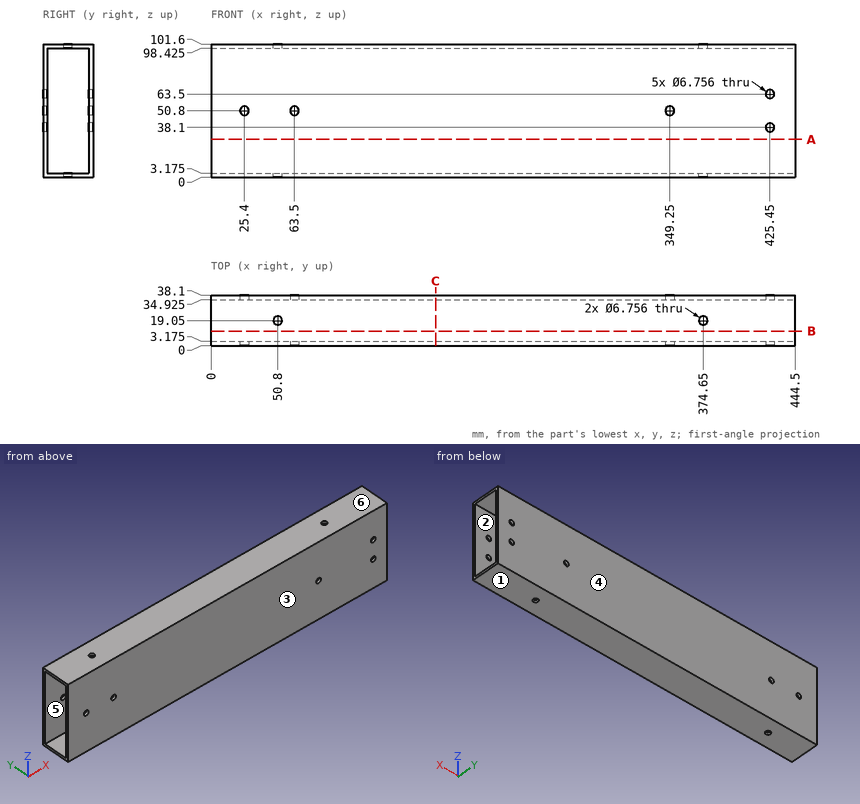
Design review of the part shown in the three views and the two pictorial views. Dimensions are in mm from the part's minimum x, y and z. A direction names the side the tool comes from. Round coordinates to 2 decimals unless told otherwise and drop trailing zeros. Write each loop counter-clockwise with the first axis right and the second up, starting at its lowest first coordinate (ties: lowest second). Pieces come first, ordered by that corner, then holes. Notation, with made-up numbers: M 20,27 L 66,27 A26 ccw 66,46 Z; hole C 21,5.5 d1. An arc over 180 degrees is marked long. Use a Markdown table: item, result. Add a question column.
Q1. To check wall thickness, follow line 1 (Z direction, x = 224.5, y = 32.5) (1 decimal); line 2 (Y direction, x = 45.5, z = 31.5) (1 decimal); line 3 (X direction, y = 2, z = 63). State the ranges of each line that lie inside material, in increasing order.
Q2. We need section B-B, the plane y = 11. State the section outline as (x, z) points (1 decimal), plus the area to 3 significant figures.
Q3. Machinability: for the marked faces 1 and 2, which of the approach directions +Z, -Z, +X, -X, +Y, -Y give a long, thin tool a straight path to every point of the face, cutting with its end or side? Answer none if there is none.
Q4. We need section A-A, the plane z = 29. State the section outline as (x, y) points (1 decimal), plus the area to 3 significant figures.
Q5. The part is to be moulded in two halves that separate along Y. For the marked faces 3, 4, 5 and 6, say which applies: pulls with the +Y half, pulls with the -Y half, needs draft (parallel to the pull), parting line crosses it, or undercut.
Q6. Insertion check: pin 1 (11 mm diameter, centred on x = 50.8, y = 19.05, fed in from -Z); pin 2 (5.5 mm diameter, centred on x = 25.4, z = 50.8, fed in from +Y). Each pin has a flat end and moves straight along its axis. Give the tip position at first contact, or say it passes through.
Q7. We need section C-C, the plane x = 171. State the section outline as (y, z) points (1 decimal).
Findings below:
| question | item | result |
|---|---|---|
| 1 | line 1 | z = 0 to 3.2, 98.4 to 101.6 |
| 1 | line 2 | y = 0 to 3.2, 34.9 to 38.1 |
| 1 | line 3 | x = 0 to 422.11, 428.79 to 444.5 |
| 2 | outline | M 0,0 L 444.5,0 L 444.5,3.2 L 0,3.2 Z; M 0,98.4 L 444.5,98.4 L 444.5,101.6 L 0,101.6 Z |
| 2 | area | 2,820 mm² |
| 3 | face 1 | -Z, +X, -X, +Y, -Y |
| 3 | face 2 | +X, -X |
| 4 | outline | M 0,0 L 444.5,0 L 444.5,3.2 L 0,3.2 Z; M 0,34.9 L 444.5,34.9 L 444.5,38.1 L 0,38.1 Z |
| 4 | area | 2,820 mm² |
| 5 | face 3 | pulls with the -Y half |
| 5 | face 4 | pulls with the +Y half |
| 5 | face 5 | undercut |
| 5 | face 6 | needs draft |
| 6 | pin 1 | stops at z = 0 |
| 6 | pin 2 | passes through |
| 7 | outline | M 0,0 L 38.1,0 L 38.1,101.6 L 0,101.6 Z; hole M 3.2,3.2 L 34.9,3.2 L 34.9,98.4 L 3.2,98.4 Z |
